from build123d import *

# Parameters (mm, degrees)
BOSS_EXTRU_1_DEPTH = 8


with BuildPart() as part:
    # Esquisse1 → Boss.-Extru.1 (new body)
    with BuildSketch(Plane(origin=(0, 0, 0), x_dir=(-1, 0, 0), z_dir=(0, 0, -1))):
        Polygon((43.918221478, 28.008066704), (2.599421562, -13.310733211), (2.599421562, -33.949941515), (66.786548928, 30.237185851), (135.349894027, 30.237185851), (199.537021393, -33.949941515), (199.537021393, -13.310733211), (158.218221478, 28.008066704), (158.218221478, 109.848159974), (138.218221478, 109.848159974), (138.218221478, 40.237185851), (63.918221478, 40.237185851), (63.918221478, 109.848159974), (43.918221478, 109.848159974), align=None)
    extrude(amount=-BOSS_EXTRU_1_DEPTH)


solid = part.part
Can you work these out from the model? Positions are in its coordinate system, mm. A direction names the side the tool comes from. Coordinates: 2 decimals unless noted, no trailing zeros. Order: outer loops, then holes, each group sorted by start corner. A loop starts at its lowest first (then second) coordinate and runs counter-clockwise, first axis right, second up. Notation, with made-up numbers: (-39.75, 50.5) - (-0.75, 50.5) arc R26 cw to (-0.75, 86.5) - close; hole circle Ø11 at (68.5, 88). An arc over 180 degrees is marked (long way). Answer as a JSON object with one key per item and string values. Group by question number.
Q1. Imagine slicing it at B-B (z = 3.5). Please give me the cut outline in (x, y), and give its area (3 significant figures).
Q2. Will these pins go through, and if not, where does the flat tip stop? P1, Ø2.5, axis at x = -84.5, z = 5.5, coming from the +Y side; P2, Ø1.5, axis at y = 77, z = 1.5, coming from the +X side; P3, Ø2, axis at x = -155, y = 21, coming from the -Z side; P4, Ø4, axis at y = -0.5, z = 2, coming from the -X side.
Q3. On a 3-axis mill with a long thin cutter (end or side, diameter ignored), from which of +Z, -Z, +X, -X, +Y, -Y can I reach the whole of each face in a straight line? I mean faces 1 (the face through (-34.24, -2.31, 3.94)), 2 (the face through (-23.55, 7.64, 3.94)), 3 (the face through (-63.918, 75, 4)), 4 (the face through (-158.218, 68, 4)), 5 (the face through (-54, 109.848, 4)). Say none if no direction works.
Q4. Imagine slicing it at C-C (y = 23). Please give me the cut outline in (x, z), and give its area (3 significant figures).
Q5. I need wall thicknesses on line 1 (X direction, y = 97.5, z = 4); line 2 (Y direction, x = -82.5, z = 1.25); line 3 (X direction, y = 30, z = 6.25). Which ranges of each line are inside material? Lowest first, please. Write a range as from..to.
Q6. Imagine slicing it at A-A (y = 50.5). Please give me the cut outline in (x, z), and give its area (3 significant figures).
Q7. Imagine slicing it at D-D (x = -85). Please give me the cut outline in (y, z), and give its area (3 significant figures).
Q8. We'd pull the mould along X, two halves only. Please class faces 6 (the face through (-179.167, 7.059, 3.944)), 7 (the face through (-102, 40.237, 4)), 8 (the face through (-43.918, 70, 4)): +X half, -X half, draft (parallel to the pull), parting line (faces both ways), or undercut.
Determined:
{
 "1": {"outline": "(-199.54, -33.95) - (-135.35, 30.24) - (-66.79, 30.24) - (-2.6, -33.95) - (-2.6, -13.31) - (-43.92, 28.01) - (-43.92, 109.85) - (-63.92, 109.85) - (-63.92, 40.24) - (-138.22, 40.24) - (-138.22, 109.85) - (-158.22, 109.85) - (-158.22, 28.01) - (-199.54, -13.31) - close", "area": "6,160 mm2"},
 "2": {"P1": "stops at y = 40.24", "P2": "stops at x = -43.92", "P3": "stops at z = 0", "P4": "stops at x = -188.73"},
 "3": {"face 1": "+Z, -Z, -Y", "face 2": "+Z, -Z, +X, +Y", "face 3": "+Z, -Z, +Y", "face 4": "+Z, -Z, -X, +Y", "face 5": "+Z, -Z, +X, -X, +Y"},
 "4": {"outline": "(-163.23, 0) - (-142.59, 0) - (-142.59, 8) - (-163.23, 8) - close; (-59.55, 0) - (-38.91, 0) - (-38.91, 8) - (-59.55, 8) - close", "area": "330 mm2"},
 "5": {"line 1": "x = -158.22..-138.22, -63.92..-43.92", "line 2": "y = 30.24..40.24", "line 3": "x = -158.22..-135.59, -66.55..-43.92"},
 "6": {"outline": "(-158.22, 0) - (-138.22, 0) - (-138.22, 8) - (-158.22, 8) - close; (-63.92, 0) - (-43.92, 0) - (-43.92, 8) - (-63.92, 8) - close", "area": "320 mm2"},
 "7": {"outline": "(30.24, 0) - (40.24, 0) - (40.24, 8) - (30.24, 8) - close", "area": "80.0 mm2"},
 "8": {"face 6": "-X half", "face 7": "undercut", "face 8": "+X half"}
}
